The listing builds one solid part. Answer for the finished solid, in the listing's coordinates (mm). Round coordinates to 2 decimals unless told otherwise and drop trailing zeros. Write each loop counter-clockwise with the first axis right and the second up, starting at its lowest first coordinate (ties: lowest second). Pieces come first, ordered by that corner, then holes. Notation, with made-up numbers: M 74.25,8 L 82.25,8 A4 cw 82.25,15 Z; hole C 44.5,-11.5 d5. An arc over 180 degrees is marked long. Write each question's results on one line, items separated by ' | '.
from build123d import *

# Parameters (mm, degrees)
SKETCH1_R           = 1
BOSS_EXTRUDE1_DEPTH = 5.5
BOSS_EXTRUDE2_DEPTH = 1
FILLET1_R           = 0.2


with BuildPart() as part:
    # Sketch1 → Boss-Extrude1 (new, symmetric)
    with BuildSketch(Plane.XY):
        Circle(SKETCH1_R)
    extrude(amount=BOSS_EXTRUDE1_DEPTH, both=True)

    # Sketch2 → Boss-Extrude2 (add, symmetric)
    with BuildSketch(Plane(origin=(0, 0, 0), x_dir=(1, 0, 0), z_dir=(0, 1, 0))):
        with BuildLine():
            Line((0, 5.5), (9, 5.5))
            ThreePointArc((9, 5.5), (9.707106781, 5.207106781), (10, 4.5))
            Line((10, 4.5), (10, 4.358898944))
            ThreePointArc((10, 4.358898944), (9.974679434, 4.135292146), (9.9, 3.923009049))
            ThreePointArc((9.9, 3.923009049), (9, 0), (9.9, -3.923009049))
            ThreePointArc((9.9, -3.923009049), (9.974679434, -4.135292146), (10, -4.358898944))
            Line((10, -4.358898944), (10, -4.5))
            ThreePointArc((10, -4.5), (9.707106781, -5.207106781), (9, -5.5))
            Line((9, -5.5), (0, -5.5))
            Line((0, -5.5), (0, -5.25))
            ThreePointArc((0, -5.25), (5.25, 0), (0, 5.25))
            Line((0, 5.25), (0, 5.5))
        make_face()
    extrude(amount=BOSS_EXTRUDE2_DEPTH, both=True)

    # Fillet1
    fillet1_edges = [part.edges().sort_by_distance(p)[0] for p in [
        (4.5, -1, 5.5),
        (9.707106781, -1, 5.207106781),
        (10, -1, 4.429449472),
        (9.974679434, -1, 4.135292146),
        (9, -1, 0),
        (9.974679434, -1, -4.135292146),
        (10, -1, -4.429449472),
        (9.707106781, -1, -5.207106781),
        (4.5, -1, -5.5),
        (4.5, 1, 5.5),
        (9.707106781, 1, 5.207106781),
        (10, 1, 4.429449472),
        (9.974679434, 1, 4.135292146),
        (9, 1, 0),
        (9.974679434, 1, -4.135292146),
        (10, 1, -4.429449472),
        (-1, 0, -5.5),
        (9.707106781, 1, -5.207106781),
        (4.5, 1, -5.5),
        (-1, 0, 5.5),
    ]]
    fillet(fillet1_edges, radius=FILLET1_R)


solid = part.part
1) Section C-C (y = 0) is taken. Determine the outline of the cut face in (x, z).
Return value:
outline: M -1,-5.3 A0.2 ccw -0.8,-5.5 L 9,-5.5 A1 ccw 10,-4.5 L 10,-4.36 A1 ccw 9.9,-3.92 A9 cw 9.9,3.92 A1 ccw 10,4.36 L 10,4.5 A1 ccw 9,5.5 L -0.8,5.5 A0.2 ccw -1,5.3 Z; hole M 1,-5.15 A5.25 ccw 1,5.15 Z
2) Section A-A (z = 0) is taken. Determine the outline of the cut face in (x, y), then the cut area to 3 significant figures.
Return value:
outline: C 0,0 d2; M 5.25,-1 L 8.8,-1 A0.2 ccw 9,-0.8 L 9,0.8 A0.2 ccw 8.8,1 L 5.25,1 Z | area: 10.6 mm²
3) Section B-B (x = 3.25) is taken. Determine the outline of the cut face in (y, z).
Return value:
outline: M -1,-5.3 A0.2 ccw -0.8,-5.5 L 0.8,-5.5 A0.2 ccw 1,-5.3 L 1,-4.12 L -1,-4.12 Z; M -1,4.12 L 1,4.12 L 1,5.3 A0.2 ccw 0.8,5.5 L -0.8,5.5 A0.2 ccw -1,5.3 Z
4) Find the intervals of material crossed by line 1 (X direction, y = -0.4, z = -2.25); line 2 (X direction, y = 0.85, z = 3.5); line 3 (Z direction, x = 3.5, y = 0.8), in increasing order.
Return value:
line 1: -0.92 to 0.92, 4.74 to 9.29 | line 2: -0.53 to 0.53, 3.91 to 9.7 | line 3: -5.5 to -3.91, 3.91 to 5.5
5) The mould has two halves that part along X. Classify faces 1 (the face through (7, -1, 0)), 2 (the face through (9.715, 0.011, 5.199)), 3 (the face through (0, -1, 0)): +X half, -X half, draft (parallel to the pull), parting line (faces both ways), or undercut.
Return value:
face 1: draft | face 2: +X half | face 3: undercut
6) Section D-D (x = 5) is taken. Determine the outline of the cut face in (y, z).
Return value:
outline: M -1,-5.3 A0.2 ccw -0.8,-5.5 L 0.8,-5.5 A0.2 ccw 1,-5.3 L 1,-1.6 L -1,-1.6 Z; M -1,1.6 L 1,1.6 L 1,5.3 A0.2 ccw 0.8,5.5 L -0.8,5.5 A0.2 ccw -1,5.3 Z
